from build123d import *

# Parameters (mm, degrees)
BOSS_EXTRUDE1_DEPTH            = 12
SKETCH41_R                     = 1.7
CUT_EXTRUDE7_DEPTH             = 18
CBORE_FOR_M3_SHCS1_D           = 3.4
CBORE_FOR_M3_SHCS1_CBORE_D     = 6.5
CBORE_FOR_M3_SHCS1_CBORE_DEPTH = 3
F_3DSKETCH3_START              = 9
F_3DSKETCH3_OUTLINE_R          = 3.25
F_3DSKETCH3_OUTLINE_R_2        = 1.7
F_3DSKETCH3_DEPTH              = 3
CUT_EXTRUDE10_DEPTH            = 15
CUT_EXTRUDE10_DEPTH_BACK       = 15
SKETCH52_R                     = 1.7
SKETCH58_R                     = 3.25
CUT_EXTRUDE11_DEPTH            = 8
CUT_EXTRUDE12_DEPTH            = 4
CUT_EXTRUDE12_DEPTH_BACK       = 6
FILLET1_R                      = 2
SKETCH61_R                     = 3.25
CUT_EXTRUDE13_DEPTH            = 6
CUT_EXTRUDE14_DEPTH            = 1


# Read off the part's stored shape, not the designer's step: 3DSketch3
with BuildPart() as part:
    # Sketch1 → Boss-Extrude1 (new body)
    with BuildSketch(Plane(origin=(0, 0, 0), x_dir=(0, 1, 0), z_dir=(0, 0, 1))):
        with BuildLine():
            Line((-6.350852961, -13), (13.279056191, -13))
            Line((13.279056191, -13), (13.279056191, -1))
            Line((13.279056191, -1), (3.97617907, -1))
            ThreePointArc((3.97617907, -1), (3.650947901, -1.865631106), (3.14, -2.636361129))
            Line((3.14, -2.636361129), (-3.14, -2.636361129))
            ThreePointArc((-3.14, -2.636361129), (-3.852531635, -1.402854233), (-4.1, 0))
            ThreePointArc((-4.1, 0), (-0.503818326, 4.06892702), (3.97617907, 1))
            Line((3.97617907, 1), (13.279056191, 1))
            Line((13.279056191, 1), (13.279056191, 13))
            Line((13.279056191, 13), (-6.350852961, 13))
            Line((-6.350852961, 13), (-13.856406461, 0))
            Line((-13.856406461, 0), (-6.350852961, -13))
        make_face()
    extrude(amount=BOSS_EXTRUDE1_DEPTH)

    # Sketch41 → Cut-Extrude7 (cut)
    with BuildSketch(Plane(origin=(0, 0, 0), x_dir=(0, 1, 0), z_dir=(0, 0, 1))):
        with Locations(Location((0, 8.6, 0), (0, 0, 270))):
            Circle(SKETCH41_R)
        with Locations(Location((0, -8.6, 0), (0, 0, 270))):
            Circle(SKETCH41_R)
    extrude(amount=CUT_EXTRUDE7_DEPTH, mode=Mode.SUBTRACT)

    # CBORE for M3 SHCS1 (through all)
    with Locations(Plane(origin=(-8.6, 0, 12), x_dir=(1, 0, 0), z_dir=(0, 0, 1))):
        with Locations((0, 0)):
            CounterBoreHole(CBORE_FOR_M3_SHCS1_D / 2, CBORE_FOR_M3_SHCS1_CBORE_D / 2, CBORE_FOR_M3_SHCS1_CBORE_DEPTH)

    # 3DSketch3 outline → 3DSketch3 (cut)
    with BuildSketch(Plane.XY.offset(F_3DSKETCH3_START)):
        with Locations((8.6, 0)):
            Circle(F_3DSKETCH3_OUTLINE_R)
        with Locations((8.6, 0)):
            Circle(F_3DSKETCH3_OUTLINE_R_2, mode=Mode.SUBTRACT)
    extrude(amount=F_3DSKETCH3_DEPTH, mode=Mode.SUBTRACT)

    # Sketch52 → Cut-Extrude10 (cut, two sides: drawn at the far end of the back side and taken through both)
    with BuildSketch(Plane.YZ.offset(-1).offset(-CUT_EXTRUDE10_DEPTH_BACK)):
        with Locations((8.106406461, 6)):
            Circle(SKETCH52_R)
    extrude(amount=CUT_EXTRUDE10_DEPTH + CUT_EXTRUDE10_DEPTH_BACK, mode=Mode.SUBTRACT)

    # Sketch58 → Cut-Extrude11 (cut)
    with BuildSketch(Plane.YZ.offset(13)):
        with Locations(Location((8.106406461, 6, 0), (0, 0, 270))):
            Circle(SKETCH58_R)
    extrude(amount=-CUT_EXTRUDE11_DEPTH, mode=Mode.SUBTRACT)

    # Sketch60 → Cut-Extrude12 (cut, two sides: drawn at the far end of the back side and taken through both)
    with BuildSketch(Plane.YZ.offset(-8).offset(-CUT_EXTRUDE12_DEPTH_BACK)):
        Polygon((8.106406461, 2.709103466), (10.956406461, 4.354551733), (10.956406461, 7.645448267), (8.106406461, 9.290896534), (5.256406461, 7.645448267), (5.256406461, 4.354551733), align=None)
    extrude(amount=CUT_EXTRUDE12_DEPTH + CUT_EXTRUDE12_DEPTH_BACK, mode=Mode.SUBTRACT)

    # Fillet1
    # the kernel refuses this fillet: 2 mm, written as the material it takes off along each edge
    with BuildSketch(Plane(origin=(13, 13.279056191, -5), x_dir=(0, -1, 0), z_dir=(0, 0, 1)), Plane(origin=(-13, 13.279056191, -5), x_dir=(1, 0, 0), z_dir=(0, 0, 1))) as fillet1_piece_1:
        with BuildLine():
            CenterArc((FILLET1_R, -FILLET1_R), FILLET1_R, 90, 90)
            Line((0, -FILLET1_R), (0, 0))
            Line((0, 0), (FILLET1_R, 0))
        make_face()
    extrude(amount=22, mode=Mode.SUBTRACT)

    # Sketch61 → Cut-Extrude13 (cut)
    with BuildSketch(Plane(origin=(0, 0, 12), x_dir=(0, 1, 0), z_dir=(0, 0, 1))):
        with Locations(Location((0, 8.6, 0), (0, 0, 270))):
            Circle(SKETCH61_R)
        with Locations(Location((0, -8.6, 0), (0, 0, 270))):
            Circle(SKETCH61_R)
    extrude(amount=-CUT_EXTRUDE13_DEPTH, mode=Mode.SUBTRACT)

    # Sketch62 → Cut-Extrude14 (cut)
    with BuildSketch(Plane(origin=(-6, -10.392304845, 0), x_dir=(-0.8660254037844386, 0.5000000000000001, 0), z_dir=(-0.5000000000000001, -0.8660254037844386, 0))):
        Polygon((0.424736725, -2.743282535), (1.346010764, -2.743282535), (1.346010764, -6.243282535), (0.897292815, -6.243282535), (0.897292815, -3.102256894), (0.134472302, -3.102256894), align=None)
    extrude(amount=-CUT_EXTRUDE14_DEPTH, mode=Mode.SUBTRACT)


solid = part.part
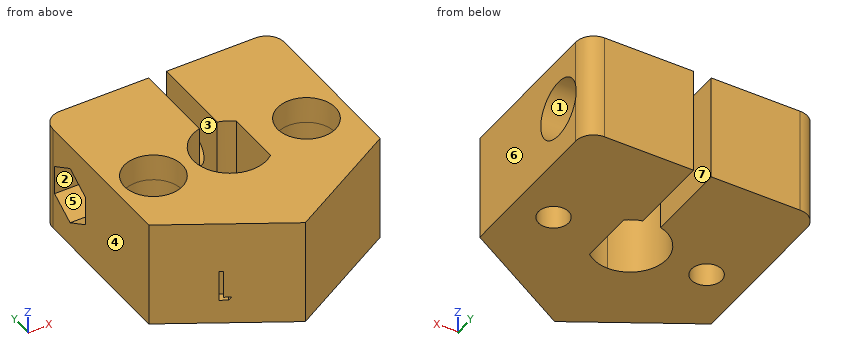
Build history of the part. All positions in model axes, mm. Face numbers are marked on the shaded views. A direction names the side the tool comes from. Round coordinates to 2 decimals unless told otherwise and drop trailing zeros. Write each loop counter-clockwise with the first axis right and the second up, starting at its lowest first coordinate (ties: lowest second). Pieces come first, ordered by that corner, then holes. Notation, with made-up numbers: (-19.75, 48) -> (-11.75, 48) arc R24 ccw to (-11.75, 78) -> close; hole circle Ø3 at (76.25, 50). An arc over 180 degrees is marked (long way). Use one line per item in the form item = value.
Q1. Tool access for the marked faces 1, 2 and 3: list every direction of +Z, -Z, +X, -X, +Y, -Y with a clear straight run to the whole face (end or side of a thin tool).
Conclusion:
face_1 = +X
face_2 = -X
face_3 = +Z, -Z, +Y
Q2. Drop flat-ended pins along their axis: P1, Ø4.5, axis at y = 8.5, z = 6, coming from the -X side; P2, Ø3, axis at y = 7.5, z = 6.5, coming from the +X side; P3, Ø3, axis at y = 7.5, z = 4, coming from the -X side; P4, Ø4, axis at x = 8.6, y = 0, coming from the +Z side. Give the stop position or say it passes through.
Conclusion:
P1 = -4
P2 = 5
P3 = -13
P4 = 6
Q3. Band-saw the part on D-D, the plane y = 5.75. Write the cut outline in (x, z), then the cut area to 3 significant figures.
Conclusion:
outline = (-13, 0) -> (-1, 0) -> (-1, 12) -> (-13, 12) -> (-13, 7.93) -> (-4, 7.93) -> (-4, 4.07) -> (-13, 4.07) -> close; (1, 0) -> (13, 0) -> (13, 3.76) -> (5, 3.76) -> (5, 8.24) -> (13, 8.24) -> (13, 12) -> (1, 12) -> close
area = 217 mm²
Q4. Drill centre lines: L1, parallel to X at y = 0, z = 4.75; L2, parallel to X at y = 10, z = 9.75; L3, parallel to Y at x = 8.6, z = 4.7. Where is each one in solid material? Low to high.
Conclusion:
L1 = -13 to -10.3, -6.9 to -4.1, 2.64 to 6.9, 10.3 to 13
L2 = -13 to -1, 1 to 13
L3 = -8.89 to -1.7, 1.7 to 5.13, 11.09 to 13.28
Q5. Two-plate mould, pull along X, no slides. Class the marked faces 4, 5, 6 and 7: released by +X, released by -X, zero draft, split by the parting line, or undercut.
Conclusion:
face_4 = released by -X
face_5 = zero draft
face_6 = released by +X
face_7 = undercut
Q6. Band-saw the part on C-C, the plane y = 0. Write the cut outline in (x, z), then the cut area to 3 significant figures.
Conclusion:
outline = (-13, 0) -> (-10.3, 0) -> (-10.3, 6) -> (-11.85, 6) -> (-11.85, 12) -> (-13, 12) -> close; (-6.9, 0) -> (-4.1, 0) -> (-4.1, 12) -> (-5.35, 12) -> (-5.35, 6) -> (-6.9, 6) -> close; (2.64, 0) -> (6.9, 0) -> (6.9, 6) -> (5.35, 6) -> (5.35, 12) -> (2.64, 12) -> close; (10.3, 0) -> (13, 0) -> (13, 12) -> (11.85, 12) -> (11.85, 6) -> (10.3, 6) -> close
area = 112 mm²
Q7. Band-saw the part on A-A, the plane z = 10.75. Write the cut outline in (x, y), then the cut area to 3 significant figures.
Conclusion:
outline = (-13, -6.35) -> (0, -13.86) -> (13, -6.35) -> (13, 11.28) arc R2 ccw to (11, 13.28) -> (1, 13.28) -> (1, 3.98) arc R4.1 cw to (2.64, 3.14) -> (2.64, -3.14) arc R4.1 cw (long way) to (-1, 3.98) -> (-1, 13.28) -> (-11, 13.28) arc R2 ccw to (-13, 11.28) -> close; hole circle Ø6.5 at (-8.6, 0); hole circle Ø6.5 at (8.6, 0)
area = 475 mm²
Q8. Band-saw the part on B-B, the plane x = -8.6. Write the cut outline in (y, z).
Conclusion:
outline = (-8.89, 0) -> (-1.7, 0) -> (-1.7, 6) -> (-3.25, 6) -> (-3.25, 12) -> (-8.89, 12) -> close; (1.7, 0) -> (13.28, 0) -> (13.28, 12) -> (3.25, 12) -> (3.25, 6) -> (1.7, 6) -> close; hole (5.26, 4.35) -> (8.11, 2.71) -> (10.96, 4.35) -> (10.96, 7.65) -> (8.11, 9.29) -> (5.26, 7.65) -> close
